Autodesk Inventor part; units mm, degrees
ref_plane "YZ Plane" through (0, 0, 0) normal (1, 0, 0) x (0, 1, 0)
ref_plane "XZ Plane" through (0, 0, 0) normal (0, 1, 0) x (-1, 0, 0)
ref_plane "XY Plane" through (0, 0, 0) normal (0, 0, 1) x (1, 0, 0)
sketch "Sketch1" plane through (0, 0, 0) normal (0, 0, 1) x (1, 0, 0)
  line L0 (25.4, -63.5) -> (-25.4, -63.5)
  line L1 (-25.4, -63.5) -> (-25.4, 63.5)
  line L2 (-25.4, 63.5) -> (25.4, 63.5)
  line L3 (25.4, 63.5) -> (25.4, -63.5)
  point P0 (0, 0)
  dimension "d0" = 50.8
  dimension "d1" = 127
  dimension "d2" = 63.5
  dimension "d3" = 25.4
extrude "Extrusion1" add sketch "Sketch1" along normal blind 6.35
sketch "Sketch2" plane through (0, 0, 6.35) normal (0, 0, 1) x (1, 0, 0)
  line L0 (25.4, -63.5) -> (25.4, 63.5)
  line L1 (25.4, 63.5) -> (-25.4, 63.5)
  line L2 (-25.4, 63.5) -> (-25.4, 57.15)
  line L3 (-25.4, 57.15) -> (25.4, 57.15)
  line L4 (25.4, 57.15) -> (25.4, 63.5)
  line L5 (25.4, -63.5) -> (-25.4, -63.5)
  line L6 (-25.4, -63.5) -> (-25.4, -57.15)
  line L7 (-25.4, -57.15) -> (25.4, -57.15)
  line L8 (25.4, -57.15) -> (25.4, -63.5)
  point P0 (0, 0)
  dimension "d6" = 50.8
  dimension "d7" = 6.35
  dimension "d8" = 50.8
  dimension "d9" = 6.35
extrude "Extrusion2" add sketch "Sketch2" along normal blind 50.8
fillet "Fillet1" radius 3.175 8 edges at (-25.4, 60.325, 57.15) (25.4, 60.325, 57.15) (-25.4, -60.325, 57.15) (25.4, -60.325, 57.15) (0, -63.5, 0) (0, 63.5, 0) (0, 57.15, 6.35) (0, -57.15, 6.35)
sketch "Sketch3" plane through (-25.4, 57.15, 9.525) normal (0, -1, 0) x (1, 0, 0)
  circle A0 centre (25.4, 38.0964) radius 3.175
  line L0 (0, -6.35) -> (0, 44.45)
  line L1 (0, -0.0036) -> (75.5058, -0.0036) construction
  point P0 (25.4, -9.525)
  dimension "d13" = 6.35
  dimension "d14" = 25.4
  dimension "d15" = 38.1
extrude "Extrusion3" add sketch "Sketch3" along normal blind 12.7
sketch "Sketch4" plane through (-25.4, -57.15, 9.525) normal (0, 1, 0) x (1, 0, 0)
  circle A0 centre (25.4, -38.1) radius 3.175
  line L0 (0, 0) -> (100.0722, 0) construction
  line L1 (0, 6.35) -> (0, -44.45) construction
  point P0 (25.4, 9.525)
  dimension "d18" = 6.35
  dimension "d19" = 38.1
  dimension "d20" = 25.4
extrude "Extrusion4" add sketch "Sketch4" along normal blind 12.7
properties part number "Bracket3"
Source: CAD feature listing. Evaluate the final solid. Frame: model axes, mm. A direction names the side the tool comes from. Coordinates: 2 decimals unless noted, no trailing zeros. Write each loop counter-clockwise with the first axis right and the second up, starting at its lowest first coordinate (ties: lowest second). Pieces come first, ordered by that corner, then holes. Notation, with made-up numbers: (15, 53.25) -> (60, 53.25) arc R20 cw to (60, 85.25) -> close; hole circle Ø5 at (37, 51). An arc over 180 degrees is marked (long way). Return JSON: item names as keys, results as strings. Group by question number.
1) Section query A-A, the plane z = 42.5. Return loops of the section in (x, y), plus the area to 3 significant figures.
2) Section query B-B, the plane x = 0. Return loops of the section in (y, z) (3 decimals).
3) Mould query, pull axis Z, two halves, no side actions, for faces 3 (the face through (0, -60, 57.15)), 4 (the face through (-0.688, -50.889, 44.526)), 5 (the face through (-0.69, 50.89, 50.72)), 6 (the face through (0, 1, 0)). Classes: +Z half, -Z half, draft (parallel to the pull), parting line (faces both ways), or undercut.
4) Contact query for flat-ended pins moving along their axis: P1, Ø1.5, axis at x = 8, y = 6, coming from the -Z side; P2, Ø15, axis at x = -5, y = 5, coming from the +Z side. Output: stop coordinate, or through.
5) Section query C-C, the plane y = 51. Return loops of the section in (x, z) (3 decimals), plus the area to 3 significant figures.
6) Ray query, line 1 along Y through (x, z) = (12, 50.5); line 2 along Z through (x, y) = (-9.5, -0.5); line 3 along Y through (x, z) = (0.5, 7). Return the intervals inside material, ascending.
7) Section query D-D, the plane y = -25.5. Return loops of the section in (x, z).
8) Set-up query: faces 1 (the face through (25.4, 0, 5)), 2 (the face through (0, -44.45, 48)). Return all of +Z, -Z, +X, -X, +Y, -Y with unobstructed straight access to the full face (end or side cutting, diameter ignored); none if empty.
From the geometry:
{
 "1": {"outline": "(-25.4, -63.5) -> (25.4, -63.5) -> (25.4, -57.15) -> (-25.4, -57.15) -> close; (-25.4, 57.15) -> (25.4, 57.15) -> (25.4, 63.5) -> (-25.4, 63.5) -> close", "area": "645 mm²"},
 "2": {"outline": "(-63.5, 3.175) arc R3.175 ccw to (-60.325, 0) -> (60.325, 0) arc R3.175 ccw to (63.5, 3.175) -> (63.5, 57.15) -> (57.15, 57.15) -> (57.15, 50.796) -> (44.45, 50.796) -> (44.45, 44.446) -> (57.15, 44.446) -> (57.15, 9.525) arc R3.175 cw to (53.975, 6.35) -> (-53.975, 6.35) arc R3.175 cw to (-57.15, 9.525) -> (-57.15, 44.45) -> (-44.45, 44.45) -> (-44.45, 50.8) -> (-57.15, 50.8) -> (-57.15, 57.15) -> (-63.5, 57.15) -> close"},
 "3": {"face 3": "+Z half", "face 4": "undercut", "face 5": "undercut", "face 6": "-Z half"},
 "4": {"P1": "z = 0", "P2": "z = 6.35"},
 "5": {"outline": "(-25.4, 0) -> (25.4, 0) -> (25.4, 6.35) -> (-25.4, 6.35) -> close; circle Ø6.35 at (0, 47.621)", "area": "354 mm²"},
 "6": {"line 1": "-63.5 to -57.15, 57.15 to 63.5", "line 2": "0 to 6.35", "line 3": "-63.5 to -55.9, 55.9 to 63.5"},
 "7": {"outline": "(-25.4, 0) -> (25.4, 0) -> (25.4, 6.35) -> (-25.4, 6.35) -> close"},
 "8": {"face 1": "+Z, -Z, +X, +Y, -Y", "face 2": "+Z, +X, -X"}
}
